```python
from build123d import *

# Parameters (mm, degrees)
SKETCH1_R           = 5
SKETCH1_R_2         = 2.5
BOSS_EXTRUDE1_DEPTH = 3.97
SKETCH2_R           = 4.35
SKETCH2_R_2         = 3.225
CUT_EXTRUDE1_DEPTH  = 0.25
SKETCH3_R           = 4.35
SKETCH3_R_2         = 3.225
CUT_EXTRUDE2_DEPTH  = 0.25


with BuildPart() as part:
    # Sketch1 → Boss-Extrude1 (new body)
    with BuildSketch(Plane(origin=(0, 0, 0), x_dir=(1, 0, 0), z_dir=(0, 1, 0))):
        Circle(SKETCH1_R)
        Circle(SKETCH1_R_2, mode=Mode.SUBTRACT)
    extrude(amount=BOSS_EXTRUDE1_DEPTH)

    # Sketch2 → Cut-Extrude1 (cut)
    with BuildSketch(Plane(origin=(0, 3.97, 0), x_dir=(1, 0, 0), z_dir=(0, 1, 0))):
        Circle(SKETCH2_R)
        Circle(SKETCH2_R_2, mode=Mode.SUBTRACT)
    extrude(amount=-CUT_EXTRUDE1_DEPTH, mode=Mode.SUBTRACT)

    # Sketch3 → Cut-Extrude2 (cut)
    with BuildSketch(Plane.XZ):
        Circle(SKETCH3_R)
        Circle(SKETCH3_R_2, mode=Mode.SUBTRACT)
    extrude(amount=-CUT_EXTRUDE2_DEPTH, mode=Mode.SUBTRACT)


solid = part.part
```
Can you work these out from the model? Positions are in its coordinate system, mm. A direction names the side the tool comes from. Round coordinates to 2 decimals unless told otherwise and drop trailing zeros. Loops run counter-clockwise (first coordinate to the right, second up) from the corner with the lowest first, then second, coordinate; pieces in that order, holes last. Notation, with made-up numbers: (12, 9) -> (18, 9) arc R20 ccw to (18, 39) -> close; hole circle Ø11 at (37.5, 19.5). An arc over 180 degrees is marked (long way). Answer in a Markdown table with one row per item.
Item 1: On a 3-axis mill with a long thin cutter (end or side, diameter ignored), from which of +Z, -Z, +X, -X, +Y, -Y can I reach the whole of each face in a straight line? I mean faces 4 (the flat face through (-3, 3.72, 2)), 5 (the cylindrical face through (-0.54, 1.96, 2.44)). Say none if no direction works.
Answer block:
| item | result |
|---|---|
| face 4 | +Y |
| face 5 | +Y, -Y |
Item 2: We'd pull the mould along Z, two halves only. Please class faces 1 (the flat face through (2, 3.97, 2)), 2 (the flat face through (-3, 0.25, -2)), 3 (the cylindrical face through (-1.08, 1.96, 4.88)): released by +Z, released by -Z, zero draft, split by the parting line, or undercut.
Answer block:
| item | result |
|---|---|
| face 1 | zero draft |
| face 2 | undercut |
| face 3 | split by the parting line |
Item 3: Will these pins go through, and if not, where does the flat tip stop? P1, Ø1.5, axis at x = 1, y = 1, coming from the +Z side; P2, Ø4, axis at x = 0, z = 0, coming from the -Y side.
Answer block:
| item | result |
|---|---|
| P1 | z = 4.99 |
| P2 | through |
Item 4: Suppose I cut it at C-C, the plane y = 1.35. List the corners of the cut face in (x, z) for me.
Answer block:
| item | result |
|---|---|
| outline | circle Ø10 at (0, 0); hole circle Ø5 at (0, 0) |
Item 5: Suppose I cut it at D-D, the plane z = -3.5. List the corners of the cut face in (x, y) for me, plus the area to 3 significant figures.
Answer block:
| item | result |
|---|---|
| outline | (-3.57, 0) -> (-2.58, 0) -> (-2.58, 0.25) -> (2.58, 0.25) -> (2.58, 0) -> (3.57, 0) -> (3.57, 3.97) -> (2.58, 3.97) -> (2.58, 3.72) -> (-2.58, 3.72) -> (-2.58, 3.97) -> (-3.57, 3.97) -> close |
| area | 25.8 mm² |
Item 6: Suppose I cut it at B-B, the plane x = 0. List the corners of the cut face in (y, z) for me (3 decimals).
Answer block:
| item | result |
|---|---|
| outline | (0, -5) -> (3.97, -5) -> (3.97, -4.35) -> (3.72, -4.35) -> (3.72, -3.225) -> (3.97, -3.225) -> (3.97, -2.5) -> (0, -2.5) -> (0, -3.225) -> (0.25, -3.225) -> (0.25, -4.35) -> (0, -4.35) -> close; (0, 2.5) -> (3.97, 2.5) -> (3.97, 3.225) -> (3.72, 3.225) -> (3.72, 4.35) -> (3.97, 4.35) -> (3.97, 5) -> (0, 5) -> (0, 4.35) -> (0.25, 4.35) -> (0.25, 3.225) -> (0, 3.225) -> close |
Item 7: If I drill on probe 1 along Z at (x, y) = (0, 3.8) (3 decimals); probe 2 along Z at (x, y) = (0, 2.95), over which ranges is the centre line in solid material (lowest first)?
Answer block:
| item | result |
|---|---|
| probe 1 | -5 to -4.35, -3.225 to -2.5, 2.5 to 3.225, 4.35 to 5 |
| probe 2 | -5 to -2.5, 2.5 to 5 |
Item 8: Suppose I cut it at A-A, the plane z = 0. List the corners of the cut face in (x, y) for me (3 decimals), plus the area to 3 significant figures.
Answer block:
| item | result |
|---|---|
| outline | (-5, 0) -> (-4.35, 0) -> (-4.35, 0.25) -> (-3.225, 0.25) -> (-3.225, 0) -> (-2.5, 0) -> (-2.5, 3.97) -> (-3.225, 3.97) -> (-3.225, 3.72) -> (-4.35, 3.72) -> (-4.35, 3.97) -> (-5, 3.97) -> close; (2.5, 0) -> (3.225, 0) -> (3.225, 0.25) -> (4.35, 0.25) -> (4.35, 0) -> (5, 0) -> (5, 3.97) -> (4.35, 3.97) -> (4.35, 3.72) -> (3.225, 3.72) -> (3.225, 3.97) -> (2.5, 3.97) -> close |
| area | 18.7 mm² |
